from build123d import *

# Parameters (mm, degrees)
DODANIE_WYCI_GNI_CIE1_DEPTH = 28
SZKIC2_R                    = 16.5
WYTNIJ_WYCI_GNI_CIE1_DEPTH  = 28
SZKIC3_R                    = 3
WYTNIJ_WYCI_GNI_CIE2_DEPTH  = 28
SZYK_KO_OWY1_COUNT          = 6
SZKIC4_R                    = 4
WYTNIJ_WYCI_GNI_CIE3_DEPTH  = 20


with BuildPart() as part:
    # Szkic1 → Dodanie-wyciągnięcie1 (new body)
    with BuildSketch(Plane.XY):
        Polygon((-18.893335163, -36.401668679), (-18.893335163, 4.598331321), (-1.893335163, 21.598331321), (24.106664837, 21.598331321), (41.106664837, 4.598331321), (41.106664837, -36.401668679), align=None)
    extrude(amount=DODANIE_WYCI_GNI_CIE1_DEPTH)

    # Szkic2 → Wytnij-wyciągnięcie1 (cut)
    with BuildSketch(Plane(origin=(0, 0, 0), x_dir=(-1, 0, 0), z_dir=(0, 0, -1))):
        with Locations((-11.106664837, -8.401668679)):
            Circle(SZKIC2_R)
    extrude(amount=-WYTNIJ_WYCI_GNI_CIE1_DEPTH, mode=Mode.SUBTRACT)

    # Szkic3 → Wytnij-wyciągnięcie2 (cut)
    with BuildSketch(Plane(origin=(0, 0, 0), x_dir=(-1, 0, 0), z_dir=(0, 0, -1))):
        with Locations((-33.606664837, -8.401668679)):
            Circle(SZKIC3_R)
    wytnij_wyci_gni_cie2 = extrude(amount=-WYTNIJ_WYCI_GNI_CIE2_DEPTH, mode=Mode.SUBTRACT)

    # Szyk kołowy1: Wytnij-wyciągnięcie2 ×6 about axis
    szyk_ko_owy1_axis = Axis((11.106664837, -8.401668679, 0), (0, 0, 1))
    for i in range(1, SZYK_KO_OWY1_COUNT):
        add(wytnij_wyci_gni_cie2.rotate(szyk_ko_owy1_axis, i * 360 / SZYK_KO_OWY1_COUNT), mode=Mode.SUBTRACT)

    # Szkic4 → Wytnij-wyciągnięcie3 (cut)
    with BuildSketch(Plane.XZ.offset(36.401668679)):
        with Locations((-10.893335163, 14)):
            Circle(SZKIC4_R)
        with Locations((33.106664837, 14)):
            Circle(SZKIC4_R)
    extrude(amount=-WYTNIJ_WYCI_GNI_CIE3_DEPTH, mode=Mode.SUBTRACT)


solid = part.part
Geometry: final body of the model. Coordinates: model frame, mm. A direction names the side the tool comes from. Give positions to 0.01 mm unless a question says otherwise; leave off trailing zeros. Write each loop counter-clockwise with the first axis right and the second up, starting at its lowest first coordinate (ties: lowest second). Pieces come first, ordered by that corner, then holes. Notation, with made-up numbers: (28, 37) -> (46, 37) arc R19 ccw to (46, 54) -> close; hole circle Ø5 at (85, 80.25). An arc over 180 degrees is marked (long way). Answer as a JSON object with one key per item and string values.
1. Ray query, probe 1 along Y at (x, z) = (21, 15.5); probe 2 along X at (y, z) = (-10, 21.5); probe 3 along X at (y, z) = (-29, 10.5). Return the intervals inside material, ascending. Write a range as from..to.
Ans:
{"probe 1": "y = -36.4..-30.56, -25.21..-21.61, 4.8..8.41, 13.76..21.6", "probe 2": "x = -18.89..-13.93, -8.85..-5.32, 27.53..31.07, 36.15..41.11", "probe 3": "x = -18.89..-12.83, -8.96..-2.93, 2.64..19.57, 25.14..31.17, 35.04..41.11"}
2. Contact query for flat-ended pins moving along their axis: pin 1 (10.5 mm diameter, centred on x = -10.89, z = 14, fed in from +Y); pin 2 (3.5 mm diameter, centred on x = -0.14, y = -27.89, fed in from -Z); pin 3 (6.5 mm diameter, centred on x = 33.5, z = 14, fed in from -Y); pin 4 (8 mm diameter, centred on x = 29.5, z = 11.5, fed in from +Y) (3 decimals). Output: stop coordinate, or through.
Ans:
{"pin 1": "stops at y = 17.85", "pin 2": "passes through", "pin 3": "stops at y = -16.4", "pin 4": "stops at y = 20.205"}
3. Cut plane D-D on x = 17.5. Output: boundary loops of the cut face in (y, z), and give its area (3 significant figures).
Ans:
{"outline": "(-36.4, 0) -> (-23.61, 0) -> (-23.61, 28) -> (-36.4, 28) -> close; (6.81, 0) -> (21.6, 0) -> (21.6, 28) -> (6.81, 28) -> close", "area": "772 mm^2"}
4. Cut plane C-C on y = -28.5. Output: boundary loops of the cut face in (x, z).
Ans:
{"outline": "(-18.89, 0) -> (-3.08, 0) -> (-3.08, 28) -> (-18.89, 28) -> close; (2.79, 0) -> (19.42, 0) -> (19.42, 28) -> (2.79, 28) -> close; (25.29, 0) -> (41.11, 0) -> (41.11, 28) -> (25.29, 28) -> close; hole circle Ø8 at (-10.89, 14); hole circle Ø8 at (33.11, 14)"}
5. Cut plane B-B on z = 14. Output: boundary loops of the cut face in (x, y), and give its area (3 significant figures).
Ans:
{"outline": "(-18.89, -36.4) -> (-14.89, -36.4) -> (-14.89, -16.4) -> (-6.89, -16.4) -> (-6.89, -36.4) -> (29.11, -36.4) -> (29.11, -16.4) -> (37.11, -16.4) -> (37.11, -36.4) -> (41.11, -36.4) -> (41.11, 4.6) -> (24.11, 21.6) -> (-1.89, 21.6) -> (-18.89, 4.6) -> close; hole circle Ø6 at (-11.39, -8.4); hole circle Ø33 at (11.11, -8.4); hole circle Ø6 at (-0.14, -27.89); hole circle Ø6 at (-0.14, 11.08); hole circle Ø6 at (22.36, -27.89); hole circle Ø6 at (22.36, 11.08); hole circle Ø6 at (33.61, -8.4)", "area": "1,850 mm^2"}
6. Cut plane A-A on x = 9. Output: boundary loops of the cut face in (y, z).
Ans:
{"outline": "(-36.4, 0) -> (-24.77, 0) -> (-24.77, 28) -> (-36.4, 28) -> close; (7.96, 0) -> (21.6, 0) -> (21.6, 28) -> (7.96, 28) -> close"}
7. Mould query, pull axis Y, two halves, no side actions, for faces 1 (the flat face through (-2, -20, 28)), 2 (the cylindrical face through (36.604, -8.27, 13.804)), 3 (the flat face through (11, 21.598, 14)). Classes: pulls with the +Y half, pulls with the -Y half, needs draft (parallel to the pull), parting line crosses it, or undercut.
Ans:
{"face 1": "needs draft", "face 2": "undercut", "face 3": "pulls with the +Y half"}
8. Access query for faces 4 (the cylindrical face through (-4.631, -3.446, 13.804)), 5 (the cylindrical face through (36.922, -26.542, 15.201)). Directions: +Z, -Z, +X, -X, +Y, -Y. A direction counts if a zero-diameter tool reaches every point of the face in a straight line with its end or side. Return the directions, or none.
Ans:
{"face 4": "+Z, -Z", "face 5": "-Y"}
